Here's how the part is built. I have some questions about the finished solid (model axes, mm). A direction names the side the tool comes from. Coordinates: 2 decimals unless noted, no trailing zeros. Write each loop counter-clockwise with the first axis right and the second up, starting at its lowest first coordinate (ties: lowest second). Pieces come first, ordered by that corner, then holes. Notation, with made-up numbers: (76.5, 23.25) -> (112.5, 23.25) arc R15 ccw to (112.5, 45.25) -> close; hole circle Ø1 at (-8, 42). An arc over 180 degrees is marked (long way). Put each result on its own line as item: value.
```python
from build123d import *

# Parameters (mm, degrees)
SKETCH1_W            = 193
SKETCH1_H            = 116.5
SKETCH1_R            = 1.75
SKETCH1_W_2          = 47
SKETCH1_H_2          = 57.5
SKETCH1_W_3          = 72
SKETCH1_H_3          = 27
SKETCH1_W_4          = 2
SKETCH1_H_4          = 55
BOSS_EXTRUDE1_DEPTH  = 6
SKETCH3_W            = 10
SKETCH3_H            = 10
BOSS_EXTRUDE3_DEPTH  = 10
FILLET1_R            = 3
SKETCH5_W            = 2
SKETCH5_H            = 55
BOSS_EXTRUDE4_DEPTH  = 6
SKETCH6_W            = 181
SKETCH6_H            = 104.5
CUT_EXTRUDE1_DEPTH   = 4
SKETCH7_W            = 1.5
SKETCH7_H            = 55
BOSS_EXTRUDE5_DEPTH  = 44.75
SKETCH8_W            = 2
SKETCH8_H            = 55
CUT_EXTRUDE2_DEPTH   = 42.25
SKETCH10_W           = 6
SKETCH10_H           = 19
CUT_EXTRUDE3_DEPTH   = 4
FILLET3_R            = 3
SKETCH12_W           = 55
SKETCH12_H           = 2
BOSS_EXTRUDE6_DEPTH  = 1.5
SKETCH14_W           = 3
SKETCH14_H           = 44.75
BOSS_EXTRUDE7_DEPTH  = 2
SKETCH15_W           = 3
SKETCH15_H           = 44.75
BOSS_EXTRUDE8_DEPTH  = 2
BOSS_EXTRUDE9_DEPTH  = 2
SKETCH17_R           = 1.25
CUT_EXTRUDE5_DEPTH   = 6
SKETCH18_W           = 20
SKETCH18_H           = 32.75
BOSS_EXTRUDE10_DEPTH = 2
SKETCH19_W           = 50
SKETCH19_H           = 37
CUT_EXTRUDE7_DEPTH   = 4


with BuildPart() as part:
    # Sketch1 → Boss-Extrude1 (new body)
    with BuildSketch(Plane(origin=(0, 0, 0), x_dir=(1, 0, 0), z_dir=(0, 1, 0))):
        with Locations((22.87983871, -17.078434096)):
            Rectangle(SKETCH1_W, SKETCH1_H)
        with Locations(Location((-31.988235573, -1.578434096, 0), (0, 0, 270))):
            Circle(SKETCH1_R, mode=Mode.SUBTRACT)
        with Locations(Location((-31.988235573, -32.578434096, 0), (0, 0, 270))):
            Circle(SKETCH1_R, mode=Mode.SUBTRACT)
        with Locations(Location((44.011764427, -1.578434096, 0), (0, 0, 270))):
            Circle(SKETCH1_R, mode=Mode.SUBTRACT)
        with Locations(Location((44.011764427, -32.578434096, 0), (0, 0, 270))):
            Circle(SKETCH1_R, mode=Mode.SUBTRACT)
        with Locations(Location((-70.62016129, -72.328434096, 0), (0, 0, 270))):
            Circle(SKETCH1_R, mode=Mode.SUBTRACT)
        with Locations(Location((-70.62016129, 38.171565904, 0), (0, 0, 270))):
            Circle(SKETCH1_R, mode=Mode.SUBTRACT)
        with Locations(Location((116.37983871, -72.328434096, 0), (0, 0, 270))):
            Circle(SKETCH1_R, mode=Mode.SUBTRACT)
        with Locations(Location((116.37983871, 38.171565904, 0), (0, 0, 270))):
            Circle(SKETCH1_R, mode=Mode.SUBTRACT)
        with Locations((80.308659112, -17.078434096)):
            Rectangle(SKETCH1_W_2, SKETCH1_H_2, mode=Mode.SUBTRACT)
        with Locations((6.011764427, -17.078434096)):
            Rectangle(SKETCH1_W_3, SKETCH1_H_3, mode=Mode.SUBTRACT)
        with Locations((-47.331266899, -17.078434096)):
            Rectangle(SKETCH1_W_4, SKETCH1_H_4, mode=Mode.SUBTRACT)
    extrude(amount=BOSS_EXTRUDE1_DEPTH)

    # Sketch3 → Boss-Extrude3 (add)
    with BuildSketch(Plane.XZ):
        with Locations((-62.62016129, 64.328434096)):
            Rectangle(SKETCH3_W, SKETCH3_H)
        with Locations((-62.62016129, -30.171565904)):
            Rectangle(SKETCH3_W, SKETCH3_H)
        with Locations((108.37983871, -30.171565904)):
            Rectangle(SKETCH3_W, SKETCH3_H)
        with Locations((108.37983871, 64.328434096)):
            Rectangle(SKETCH3_W, SKETCH3_H)
    extrude(amount=BOSS_EXTRUDE3_DEPTH)

    # Fillet1
    fillet1_edges = [part.edges().sort_by_distance(p)[0] for p in [
        (56.808659112, 3, -11.671565904),
        (56.808659112, 3, 45.828434096),
        (103.808659112, 3, 45.828434096),
        (103.808659112, 3, -11.671565904),
    ]]
    fillet(fillet1_edges, radius=FILLET1_R)

    # Sketch5 → Boss-Extrude4 (add)
    with BuildSketch(Plane.XZ):
        with Locations((-47.331266899, 17.078434096)):
            Rectangle(SKETCH5_W, SKETCH5_H)
    extrude(amount=-BOSS_EXTRUDE4_DEPTH)

    # Sketch6 → Cut-Extrude1 (cut)
    with BuildSketch(Plane.XZ.offset(10)):
        with Locations((22.87983871, 17.078434096)):
            Rectangle(SKETCH6_W, SKETCH6_H)
    extrude(amount=-CUT_EXTRUDE1_DEPTH, mode=Mode.SUBTRACT)

    # Sketch7 → Boss-Extrude5 (add)
    with BuildSketch(Plane.XZ):
        with Locations((-61.87016129, 17.078434096)):
            Rectangle(SKETCH7_W, SKETCH7_H)
    extrude(amount=BOSS_EXTRUDE5_DEPTH)

    # Sketch8 → Cut-Extrude2 (cut)
    with BuildSketch(Plane.XZ):
        with Locations((-60.12016129, 17.078434096)):
            Rectangle(SKETCH8_W, SKETCH8_H)
    extrude(amount=-CUT_EXTRUDE2_DEPTH, mode=Mode.SUBTRACT)

    # Sketch10 → Cut-Extrude3 (cut)
    with BuildSketch(Plane.XZ):
        with Locations((45.011764427, 17.078434096)):
            Rectangle(SKETCH10_W, SKETCH10_H)
    extrude(amount=-CUT_EXTRUDE3_DEPTH, mode=Mode.SUBTRACT)

    # Fillet3
    fillet3_edges = [part.edges().sort_by_distance(p)[0] for p in [
        (-67.62016129, -6, 64.328434096),
        (-67.62016129, -6, -30.171565904),
        (-62.62016129, -6, -35.171565904),
        (108.37983871, -6, -35.171565904),
        (-62.62016129, -6, 69.328434096),
        (108.37983871, -6, 69.328434096),
        (113.37983871, -6, -30.171565904),
        (113.37983871, -6, 64.328434096),
        (-62.62016129, -6, 59.328434096),
        (-57.62016129, -6, 64.328434096),
        (103.37983871, -6, 64.328434096),
        (108.37983871, -6, 59.328434096),
        (108.37983871, -6, -25.171565904),
        (103.37983871, -6, -30.171565904),
        (-57.62016129, -6, -30.171565904),
        (-62.62016129, -6, -25.171565904),
    ]]
    fillet(fillet3_edges, radius=FILLET3_R)

    # Sketch12 → Boss-Extrude6 (add)
    with BuildSketch(Plane(origin=(-61.12016129, 0, 0), x_dir=(0, 0, -1), z_dir=(1, 0, 0))):
        with Locations((-17.078434096, -43.75)):
            Rectangle(SKETCH12_W, SKETCH12_H)
    extrude(amount=BOSS_EXTRUDE6_DEPTH)

    # Sketch14 → Boss-Extrude7 (add)
    with BuildSketch(Plane(origin=(0, 0, -10.421565904), x_dir=(-1, 0, 0), z_dir=(0, 0, -1))):
        with Locations((61.12016129, -22.375)):
            Rectangle(SKETCH14_W, SKETCH14_H)
    extrude(amount=BOSS_EXTRUDE7_DEPTH)

    # Sketch15 → Boss-Extrude8 (add)
    with BuildSketch(Plane.XY.offset(44.578434096)):
        with Locations((-61.12016129, -22.375)):
            Rectangle(SKETCH15_W, SKETCH15_H)
    extrude(amount=BOSS_EXTRUDE8_DEPTH)

    # Sketch16 → Boss-Extrude9 (add)
    with BuildSketch(Plane.ZY.offset(62.62016129)):
        Polygon((-10.421565904, 0), (-10.421565904, -42.75), (46.578434096, -42.75), (46.578434096, -44.75), (-12.421565904, -44.75), (-12.421565904, 0), align=None)
    extrude(amount=BOSS_EXTRUDE9_DEPTH)

    # Sketch17 → Cut-Extrude5 (cut)
    with BuildSketch(Plane(origin=(0, 6, 0), x_dir=(1, 0, 0), z_dir=(0, 1, 0))):
        with Locations(Location((57.308659112, 12.671565904, 0), (0, 0, 270))):
            Circle(SKETCH17_R)
        with Locations(Location((103.308659112, 12.671565904, 0), (0, 0, 270))):
            Circle(SKETCH17_R)
        with Locations(Location((57.308659112, -46.828434096, 0), (0, 0, 270))):
            Circle(SKETCH17_R)
        with Locations(Location((103.308659112, -46.828434096, 0), (0, 0, 270))):
            Circle(SKETCH17_R)
    extrude(amount=-CUT_EXTRUDE5_DEPTH, mode=Mode.SUBTRACT)

    # Sketch18 → Boss-Extrude10 (add)
    with BuildSketch(Plane(origin=(-59.62016129, 0, 0), x_dir=(0, 0, -1), z_dir=(1, 0, 0))):
        with Locations((-36.578434096, -16.375)):
            Rectangle(SKETCH18_W, SKETCH18_H)
        with Locations((2.421565904, -16.375)):
            Rectangle(SKETCH18_W, SKETCH18_H)
    extrude(amount=BOSS_EXTRUDE10_DEPTH)

    # Sketch19 → Cut-Extrude7 (cut)
    with BuildSketch(Plane.XZ):
        with Locations((-3.238235573, 17.078434096)):
            Rectangle(SKETCH19_W, SKETCH19_H)
    extrude(amount=-CUT_EXTRUDE7_DEPTH, mode=Mode.SUBTRACT)


solid = part.part
```
Item 1: For P1, Ø5.5, axis at x = -31.99, z = 1.58, coming from the -Y side; P2, Ø3, axis at x = 108.5, z = 65, coming from the -Y side; P3, Ø1, axis at x = -58.5, y = -20.5, coming from the +Z side; P4, Ø1, axis at x = 3.5, z = 29.5, coming from the -Y side, each with a flat end and sliding along its axis, tell me the tip position at first contact or that it passes through.
Output:
P1: stops at y = 0
P2: stops at y = -6
P3: stops at z = 46.58
P4: passes through
Item 2: Imagine slicing it at B-B on z = -6. Write out the boundary of the cut face in (x, y), then the cut area to 3 significant figures.
Output:
outline: (-73.62, 0) -> (-62.62, 0) -> (-62.62, -42.75) -> (-64.62, -42.75) -> (-64.62, -44.75) -> (-59.62, -44.75) -> (-59.62, -42.75) -> (-61.12, -42.75) -> (-61.12, 6) -> (-73.62, 6) -> close; (-59.62, -32.75) -> (-57.62, -32.75) -> (-57.62, 0) -> (56.81, 0) -> (56.81, 6) -> (-59.12, 6) -> (-59.12, 0) -> (-59.62, 0) -> close; (103.81, 0) -> (119.38, 0) -> (119.38, 6) -> (103.81, 6) -> close
area: 1,000 mm²
Item 3: Which directions (+Z, -Z, +X, -X, +Y, -Y) give clear straight access to the entire face, cutting with the end or side of a thin tool? Please do faces 1 (the flat face through (-61, -23, -12.422)), 2 (the flat face through (-59.62, -16, -1)), 3 (the flat face through (-63, -6, -30)), 4 (the flat face through (21.762, 2, 1)).
Output:
face 1: +X, -X, -Y
face 2: +Y
face 3: -Z, +X, -X, -Y
face 4: -Y
Item 4: Imagine slicing it at C-C on y = -30.5. Write out the boundary of the cut face in (x, z).
Output:
outline: (-64.62, -12.42) -> (-57.62, -12.42) -> (-57.62, 7.58) -> (-59.62, 7.58) -> (-59.62, -10.42) -> (-61.12, -10.42) -> (-61.12, 44.58) -> (-59.62, 44.58) -> (-59.62, 26.58) -> (-57.62, 26.58) -> (-57.62, 46.58) -> (-62.62, 46.58) -> (-62.62, -10.42) -> (-64.62, -10.42) -> close
Item 5: Imagine slicing it at A-A on x = 25. Write out the boundary of the cut face in (y, z), then the cut area to 3 significant figures.
Output:
outline: (0, -41.17) -> (6, -41.17) -> (6, 3.58) -> (0, 3.58) -> close; (0, 30.58) -> (6, 30.58) -> (6, 75.33) -> (0, 75.33) -> close
area: 537 mm²
Item 6: Imagine slicing it at D-D on z = 10. Write out the boundary of the cut face in (x, y), then the cut area to 3 significant figures.
Output:
outline: (-73.62, 0) -> (-62.62, 0) -> (-62.62, -42.75) -> (-64.62, -42.75) -> (-64.62, -44.75) -> (-59.62, -44.75) -> (-59.62, -42.75) -> (-61.12, -42.75) -> (-61.12, 6) -> (-73.62, 6) -> close; (-59.12, 0) -> (-29.99, 0) -> (-29.99, 6) -> (-59.12, 6) -> close; (42.01, 4) -> (48.01, 4) -> (48.01, 0) -> (56.81, 0) -> (56.81, 6) -> (42.01, 6) -> close; (103.81, 0) -> (119.38, 0) -> (119.38, 6) -> (103.81, 6) -> close
area: 482 mm²
Item 7: Please list where these lines run through material, in increasing order: line 1 along X through (y, z) = (-24, 35.5); line 2 along X through (y, z) = (2.5, 71); line 3 along Y through (x, z) = (-35.5, -7.5). Write a range as from..to.
Output:
line 1: x = -62.62..-61.12, -59.62..-57.62
line 2: x = -73.62..-71.76, -69.48..115.24, 117.52..119.38
line 3: y = 0..6
Item 8: If we mould it in two halves opening along X, with no side actions, what happens to faces 5 (the cylindrical face through (117.855, 2.958, -37.231)), 6 (the cylindrical face through (118.115, 2.958, 72.101)), 7 (the flat face through (-73.62, 3, 18)), 8 (the flat face through (-63, -6, 64))? For each: released by +X, released by -X, zero draft, split by the parting line, or undercut.
Output:
face 5: undercut
face 6: undercut
face 7: released by -X
face 8: zero draft
